Design review of the part built by this model. Coordinates are the model's own, in mm. A direction names the side the tool comes from. Coordinates: 2 decimals unless noted, no trailing zeros. Order: outer loops, then holes, each group sorted by start corner. A loop starts at its lowest first (then second) coordinate and runs counter-clockwise, first axis right, second up. Notation, with made-up numbers: (17, 5.25) - (24, 5.25) arc R14 cw to (24, 16.25) - close; hole circle Ø9 at (-20.75, 23). An arc over 180 degrees is marked (long way). Write each question's results on one line, items separated by ' | '. Start each with the question number.
```python
from build123d import *

# Parameters (mm, degrees)
F0_R     = 101.6
F1_DEPTH = 6.35
F2_R     = 25.4
F3_DEPTH = 15.875
F5_DEPTH = 22.226


with BuildPart() as f1:
    # F0 (on Top) → F1 (new body)
    with BuildSketch(Plane.XY):
        Circle(F0_R)
    extrude(amount=F1_DEPTH)

    # F2 (on face) → F3 (join)
    with BuildSketch(Plane.XY.offset(6.35)):
        Circle(F2_R)
    extrude(amount=F3_DEPTH)

    # F4 (on face) → F5 (cut, through all)
    with BuildSketch(Plane.XY.offset(22.225)):
        with BuildLine():
            ThreePointArc((-3.175, 12.296722), (-7.77713, -10.040232), (12.7, 0))
            ThreePointArc((12.7, 0), (10.040232, 7.77713), (3.175, 12.296722))
            Line((3.175, 12.296722), (3.175, 9.525))
            Line((3.175, 9.525), (-3.175, 9.525))
            Line((-3.175, 9.525), (-3.175, 12.296722))
        make_face()
        with BuildLine():
            Line((3.175, 9.525), (3.175, 12.296722))
            ThreePointArc((3.175, 12.296722), (0, 12.7), (-3.175, 12.296722))
            Line((-3.175, 12.296722), (-3.175, 9.525))
            Line((-3.175, 9.525), (3.175, 9.525))
        make_face()
        with BuildLine():
            ThreePointArc((-3.175, 12.296722), (0, 12.7), (3.175, 12.296722))
            Line((3.175, 12.296722), (3.175, 15.875))
            Line((3.175, 15.875), (-3.175, 15.875))
            Line((-3.175, 15.875), (-3.175, 12.296722))
        make_face()
    extrude(amount=-F5_DEPTH, mode=Mode.SUBTRACT)


solid = f1.part
```
(1) To check wall thickness, follow line 1 along Y through (x, z) = (0, 9.75) (3 decimals); line 2 along Y through (x, z) = (0, 5.75) (3 decimals); line 3 along Z through (x, y) = (-64.5, -43). State the ranges of each line that lie inside material, in increasing order. Write a range as [from, to].
(2) Mouldability with a two-part tool opening along X and no side actions: class faces 1 (the face through (21, 1, 0)), 2 (the face through (-22.025, -99.184, 3.131)), 3 (the face through (0, 15.875, 11)) as +X half, -X half, draft (parallel to the pull), parting line (faces both ways), or undercut.
(3) Take a section at A-A (x = 0). State the section outline as (y, z) points (3 decimals).
(4) Take a section at B-B (z = 14.5). State the section outline as (x, y) points (3 decimals), plus the area to 3 significant figures.
(5) Take a section at D-D (x = 65.5). State the section outline as (y, z) points, plus the area to 3 significant figures.
(6) Clearance check with flat-ended pins moving along their axes: pin 1 (5 mm diameter, centred on x = -1, z = 9, fed in from -Y); pin 2 (1 mm diameter, centred on x = 72.5, z = 5, fed in from +Y); pin 3 (1.1 mm diameter, centred on y = 13.5, z = 9.5, fed in from -X); pin 4 (23 mm diameter, centred on x = 0, y = 0, fed in from -Z). State where each tip first meets the part, or that it passes through.
(7) Take a section at C-C (y = 51.5). State the section outline as (x, z) points, plus the area to 3 significant figures.
(8) Tool access review of faces 4 (the face through (-5.506, -24.796, 14.176)), 5 (the face through (5, 12, 22.225)): name each direction out of +Z, -Z, +X, -X, +Y, -Y from which nothing blocks a thin tool from reaching the whole face with its end or side.
Worked out:
1) line 1: [-25.4, -12.7], [15.875, 25.4] | line 2: [-101.6, -12.7], [15.875, 101.6] | line 3: [0, 6.35]
2) face 1: draft | face 2: parting line | face 3: undercut
3) outline: (-101.6, 0) - (-12.7, 0) - (-12.7, 22.225) - (-25.4, 22.225) - (-25.4, 6.35) - (-101.6, 6.35) - close; (15.875, 0) - (101.6, 0) - (101.6, 6.35) - (25.4, 6.35) - (25.4, 22.225) - (15.875, 22.225) - close
4) outline: circle Ø50.8 at (0, 0); hole (-3.175, 12.297) arc R12.7 ccw (long way) to (12.7, 0) arc R12.7 ccw to (3.175, 12.297) - (3.175, 15.875) - (-3.175, 15.875) - close | area: 1,500 mm^2
5) outline: (-77.67, 0) - (77.67, 0) - (77.67, 6.35) - (-77.67, 6.35) - close | area: 986 mm^2
6) pin 1: y = -25.4 | pin 2: y = 71.68 | pin 3: x = -21.85 | pin 4: through
7) outline: (-87.58, 0) - (87.58, 0) - (87.58, 6.35) - (-87.58, 6.35) - close | area: 1,110 mm^2
8) face 4: +Z | face 5: +Z, +X, -X, +Y, -Y
